Could you check a few things on this drawing? It's one solid part, dimensions in mm from its lowest x, y, z. A direction names the side the tool comes from. Give positions to 0.01 mm unless a question says otherwise; leave off trailing zeros. Order: outer loops, then holes, each group sorted by start corner. A loop starts at its lowest first (then second) coordinate and runs counter-clockwise, first axis right, second up.
(1) If I drill on probe 1 along Y at (x, z) = (50.8, 48.6); probe 2 along Z at (x, y) = (27.5, 24.25); probe 3 along Y at (x, z) = (50.8, 2.1), over which ranges is the centre line in solid material (lowest first)?
(2) On a 3-axis mill with a long thin cutter (end or side, diameter ignored), from which of +Z, -Z, +X, -X, +Y, -Y can I reach the whole of each face in a straight line? I mean the marked faces 5 and 6. Say none if no direction works.
(3) If we mould it in two halves opening along Z, with no side actions, what happens to the marked faces 1, 2, 3 and 4? For each: released by +Z, released by -Z, zero draft, split by the parting line, or undercut.
(4) Imagine slicing it at B-B, the plane z = 24. Write out the boundary of the cut face in (x, y).
(5) Will these pins go through, and if not, where does the flat tip stop? pin 1 (3 mm diameter, centred on y = 1, z = 14.5, fed in from -X); pin 2 (1 mm diameter, centred on x = 138, z = 25, fed in from +Y).
(6) Imagine slicing it at A-A, the plane x = 166.5. Write out the boundary of the cut face in (y, z).
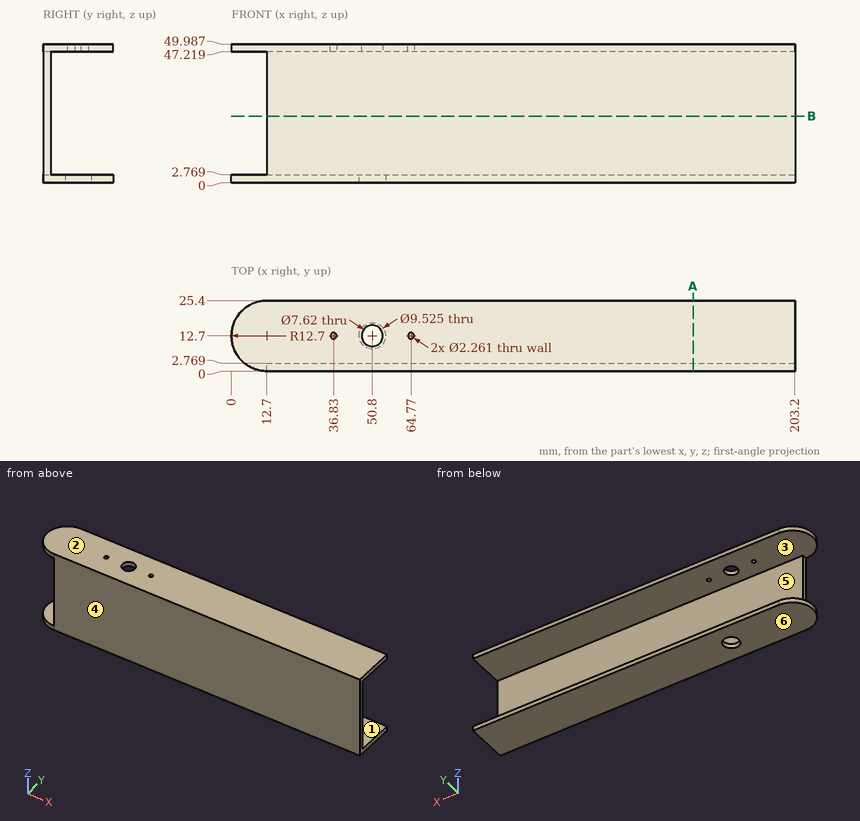
Answer block:
1. probe 1: y = 0 to 8.89, 16.51 to 25.4
1. probe 2: z = 0 to 2.77, 47.22 to 49.99
1. probe 3: y = 0 to 7.94, 17.46 to 25.4
2. face 5: +X, -X, +Y
2. face 6: -Z, +X, -X, +Y, -Y
3. face 1: undercut
3. face 2: released by +Z
3. face 3: undercut
3. face 4: zero draft
4. outline: (12.7, 0) - (203.2, 0) - (203.2, 2.77) - (12.7, 2.77) - close
5. pin 1: stops at x = 12.7
5. pin 2: stops at y = 2.77
6. outline: (0, 0) - (25.4, 0) - (25.4, 2.77) - (2.77, 2.77) - (2.77, 47.22) - (25.4, 47.22) - (25.4, 49.99) - (0, 49.99) - close
